```python
from build123d import *

# Parameters (mm, degrees)
BOSS_EXTRUDE1_DEPTH = 6
SKETCH2_R           = 1.5
CUT_EXTRUDE1_DEPTH  = 2
FILLET1_R           = 2
SKETCH3_R           = 3.5
CUT_EXTRUDE2_DEPTH  = 8
FILLET2_R           = 1


with BuildPart() as part:
    # Sketch1 → Boss-Extrude1 (new body)
    with BuildSketch(Plane.XY):
        Polygon((-24.5, 2), (-24.5, 0), (-17.5, 0), (-17.5, 37), (0, 37), (0, 39), (-19.5, 39), (-19.5, 2), align=None)
        Polygon((0, 39), (0, 37), (17.5, 37), (17.5, 0), (24.5, 0), (24.5, 2), (19.5, 2), (19.5, 39), align=None)
    extrude(amount=BOSS_EXTRUDE1_DEPTH)

    # Sketch2 → Cut-Extrude1 (cut)
    with BuildSketch(Plane(origin=(0, 2, 0), x_dir=(1, 0, 0), z_dir=(0, 1, 0))):
        with Locations(Location((-22, -3, 0), (0, 0, 180))):
            Circle(SKETCH2_R)
        with Locations((22, -3)):
            Circle(SKETCH2_R)
    extrude(amount=-CUT_EXTRUDE1_DEPTH, mode=Mode.SUBTRACT)

    # Fillet1
    fillet1_edges = [part.edges().sort_by_distance(p)[0] for p in [
        (-19.5, 39, 3),
        (19.5, 39, 3),
    ]]
    fillet(fillet1_edges, radius=FILLET1_R)

    # Sketch3 → Cut-Extrude2 (cut)
    with BuildSketch(Plane(origin=(0, 2, 0), x_dir=(1, 0, 0), z_dir=(0, 1, 0))):
        with Locations((-22, -3)):
            Circle(SKETCH3_R)
        with Locations((22, -3)):
            Circle(SKETCH3_R)
    extrude(amount=CUT_EXTRUDE2_DEPTH, mode=Mode.SUBTRACT)

    # Fillet2
    # the kernel refuses this fillet: 1 mm, written as the material it takes off along each edge
    with BuildSketch(Plane(origin=(19.5, 2, 0), x_dir=(0, 0, 1), z_dir=(0, 1, 0)), Plane(origin=(19.5, 2, 6), x_dir=(-1, 0, 0), z_dir=(0, 1, 0)), Plane(origin=(17.5, 39, 0), x_dir=(0, 0, 1), z_dir=(-1, 0, 0)), Plane(origin=(-17.5, 39, 6), x_dir=(0, 0, -1), z_dir=(1, 0, 0)), Plane(origin=(-19.5, 37, 6), x_dir=(1, 0, 0), z_dir=(0, -1, 0)), Plane(origin=(-19.5, 37, 0), x_dir=(0, 0, 1), z_dir=(0, -1, 0))) as fillet2_piece_1:
        with BuildLine():
            CenterArc((FILLET2_R, -FILLET2_R), FILLET2_R, 90, 90)
            Line((0, -FILLET2_R), (0, 0))
            Line((0, 0), (FILLET2_R, 0))
        make_face()
    extrude(amount=35, mode=Mode.SUBTRACT)
    with BuildSketch(Plane(origin=(17.5, 37, 6), x_dir=(0, 1, 0), z_dir=(-1, 0, 0))) as fillet2_piece_2:
        with BuildLine():
            CenterArc((2 - FILLET2_R, FILLET2_R), FILLET2_R, 270, 90)
            Line((2, FILLET2_R), (2, 0))
            Line((2, 0), (2 - FILLET2_R, 0))
        make_face()
    revolve(axis=Axis((17.5, 37, 6), (0, 0, -1)), revolution_arc=90, mode=Mode.SUBTRACT)
    with BuildSketch(Plane(origin=(17.5, 37, 0), x_dir=(0, 1, 0), z_dir=(-1, 0, 0))) as fillet2_piece_3:
        with BuildLine():
            CenterArc((2 - FILLET2_R, -FILLET2_R), FILLET2_R, 0, 90)
            Line((2 - FILLET2_R, 0), (2, 0))
            Line((2, 0), (2, -FILLET2_R))
        make_face()
    revolve(axis=Axis((17.5, 37, 0), (0, 0, -1)), revolution_arc=90, mode=Mode.SUBTRACT)
    with BuildSketch(Plane(origin=(-17.5, 37, 6), x_dir=(0, 1, 0), z_dir=(1, 0, 0))) as fillet2_piece_4:
        with BuildLine():
            CenterArc((2 - FILLET2_R, -FILLET2_R), FILLET2_R, 0, 90)
            Line((2, -FILLET2_R), (2, 0))
            Line((2, 0), (2 - FILLET2_R, 0))
        make_face()
    revolve(axis=Axis((-17.5, 37, 6), (0, 0, 1)), revolution_arc=90, mode=Mode.SUBTRACT)
    with BuildSketch(Plane(origin=(-17.5, 37, 0), x_dir=(0, 1, 0), z_dir=(1, 0, 0))) as fillet2_piece_5:
        with BuildLine():
            CenterArc((2 - FILLET2_R, FILLET2_R), FILLET2_R, 270, 90)
            Line((2 - FILLET2_R, 0), (2, 0))
            Line((2, 0), (2, FILLET2_R))
        make_face()
    revolve(axis=Axis((-17.5, 37, 0), (0, 0, 1)), revolution_arc=90, mode=Mode.SUBTRACT)
    with BuildSketch(Plane(origin=(24.5, -2.5, 0), x_dir=(0, 0, 1), z_dir=(0, 1, 0)), Plane(origin=(24.5, -2.5, 6), x_dir=(-1, 0, 0), z_dir=(0, 1, 0)), Plane(origin=(-24.5, 4.5, 0), x_dir=(0, 0, 1), z_dir=(0, -1, 0)), Plane(origin=(-24.5, 4.5, 6), x_dir=(1, 0, 0), z_dir=(0, -1, 0))) as fillet2_piece_6:
        with BuildLine():
            CenterArc((FILLET2_R, -FILLET2_R), FILLET2_R, 90, 90)
            Line((0, -FILLET2_R), (0, 0))
            Line((0, 0), (FILLET2_R, 0))
        make_face()
    extrude(amount=7, mode=Mode.SUBTRACT)


solid = part.part
```
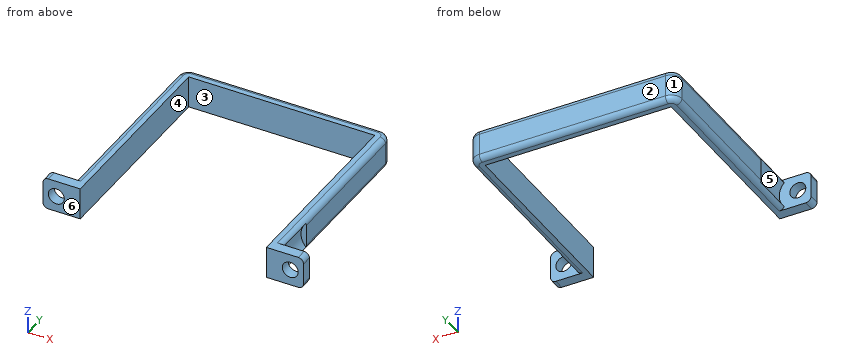
Here's how the part is built. I have some questions about the finished solid (model axes, mm). Face numbers are marked on the shaded views. A direction names the side the tool comes from. Coordinates: 2 decimals unless noted, no trailing zeros. Write each loop counter-clockwise with the first axis right and the second up, starting at its lowest first coordinate (ties: lowest second). Pieces come first, ordered by that corner, then holes. Notation, with made-up numbers: (-12.75, 46) - (16.25, 46) arc R31 ccw to (16.25, 70) - close; hole circle Ø1 at (-33, -1). An arc over 180 degrees is marked (long way). One line per item, written item: value.
1) I'm going to push flat-ended pins straight in: P1, Ø10, axis at x = 8, y = 5, coming from the -Z side; P2, Ø1.8, axis at y = 17.5, z = 3, coming from the +X side; P3, Ø3, axis at x = -20.5, z = 3.5, coming from the +Y side; P4, Ø2, axis at y = 18.5, z = 4, coming from the -X side. Where does each tip first touch, or does it pass through?
Model answer:
P1: passes through
P2: stops at x = 19.5
P3: stops at y = 38.32
P4: stops at x = -19.5
2) On a 3-axis mill with a long thin cutter (end or side, diameter ignored), from which of +Z, -Z, +X, -X, +Y, -Y can I reach the whole of each face in a straight line? I mean the marked faces 4, 5 and 6. Say none if no direction works.
Model answer:
face 4: +Z, -Z, -Y
face 5: -X
face 6: +Z, -Z, +X, -X, -Y
3) I need wall thicknesses on line 1 along X through (y, z) = (20, 1.3); line 2 along Z through (x, y) = (22, 1); line 3 along Y through (x, z) = (-2, 4.9). Which ranges of each line are inside material? Lowest first, please.
Model answer:
line 1: x = -19.5 to -17.5, 17.5 to 19.5
line 2: z = 0 to 1.5, 4.5 to 6
line 3: y = 37 to 39
4) Suppose I cut it at B-B on z = 3. Write out the boundary of the cut face in (x, y), and give its area (3 significant figures).
Model answer:
outline: (-24.5, 0) - (-23.5, 0) - (-23.5, 2) - (-24.5, 2) - close; (-20.5, 0) - (-17.5, 0) - (-17.5, 37) - (17.5, 37) - (17.5, 0) - (20.5, 0) - (20.5, 2) - (18.5, 2) - (18.5, 10) - (19.5, 10) - (19.5, 37) arc R2 ccw to (17.5, 39) - (-17.5, 39) arc R2 ccw to (-19.5, 37) - (-19.5, 10) - (-18.5, 10) - (-18.5, 2) - (-20.5, 2) - close; (23.5, 0) - (24.5, 0) - (24.5, 2) - (23.5, 2) - close
area: 216 mm²
5) Suppose I cut it at D-D on y = 18.5. Write out the boundary of the cut face in (x, z).
Model answer:
outline: (-19.5, 1) arc R1 ccw to (-18.5, 0) - (-17.5, 0) - (-17.5, 6) - (-18.5, 6) arc R1 ccw to (-19.5, 5) - close; (17.5, 0) - (18.5, 0) arc R1 ccw to (19.5, 1) - (19.5, 5) arc R1 ccw to (18.5, 6) - (17.5, 6) - close
6) We'd pull the mould along X, two halves only. Please class the marked faces 1, 2 and 3: pulls with the +X half, pulls with the -X half, needs draft (parallel to the pull), parting line crosses it, or undercut.
Model answer:
face 1: pulls with the -X half
face 2: needs draft
face 3: undercut
7) Suppose I cut it at C-C on x = -22. Write out the boundary of the cut face in (y, z), and give its area (3 significant figures).
Model answer:
outline: (0, 0) - (2, 0) - (2, 1.5) - (0, 1.5) - close; (0, 4.5) - (2, 4.5) - (2, 6) - (0, 6) - close
area: 6.00 mm²
8) Suppose I cut it at A-A on y = 7. Write out the boundary of the cut face in (x, z), and give its area (3 significant figures).
Model answer:
outline: (-19.43, 0.63) arc R1 ccw to (-18.5, 0) - (-17.5, 0) - (-17.5, 6) - (-18.5, 6) arc R1 ccw to (-19.43, 5.37) arc R3.5 cw to start; (17.5, 0) - (18.5, 0) arc R1 ccw to (19.43, 0.63) arc R3.5 cw to (19.43, 5.37) arc R1 ccw to (18.5, 6) - (17.5, 6) - close
area: 16.4 mm²
